Verification items for the finished model (mm, model axes). Face numbers are marked on the shaded views. Coordinates: 2 decimals unless noted, no trailing zeros. Order: outer loops, then holes, each group sorted by start corner. A loop starts at its lowest first (then second) coordinate and runs counter-clockwise, first axis right, second up. Notation, with made-up numbers: (-10.5, -21.75) -> (34.5, -21.75) arc R18 ccw to (34.5, -17.75) -> close; hole circle Ø5 at (2.25, -5.75). An arc over 180 degrees is marked (long way). Write item = value, one per line. Start each with the question number.
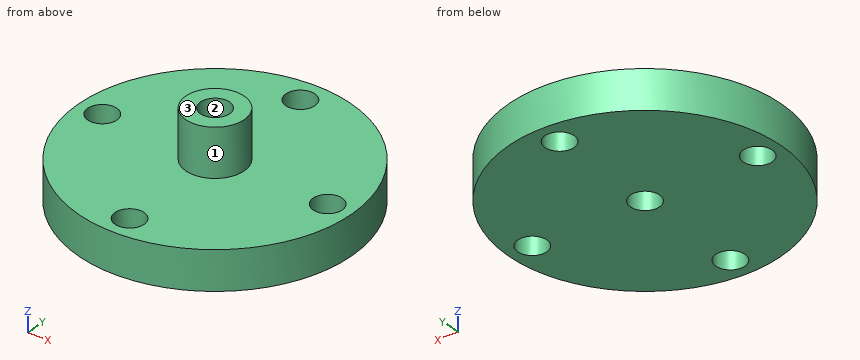
from build123d import *

# Parameters (mm, degrees)
SKETCH003_R   = 1.5
PAD003_DEPTH  = 8.9
SKETCH002_R   = 3
PAD002_DEPTH  = 4.9
SKETCH001_R   = 14
SKETCH001_R_2 = 1.5
PAD001_DEPTH  = 4


with BuildPart() as body003:
    # Sketch003 → Pad003 (new body)
    with BuildSketch(Plane.XY):
        Circle(SKETCH003_R)
    extrude(amount=PAD003_DEPTH)


with BuildPart() as body002:
    # Sketch002 (on DatumPlane) → Pad002 (new body)
    with BuildSketch(Plane.XY.offset(4)):
        Circle(SKETCH002_R)
    extrude(amount=PAD002_DEPTH)


with BuildPart() as cut:
    # Sketch001 → Pad001 (new body)
    with BuildSketch(Plane.XY):
        Circle(SKETCH001_R)
        with Locations((-11.5, 0)):
            Circle(SKETCH001_R_2, mode=Mode.SUBTRACT)
        with Locations((11.5, 0)):
            Circle(SKETCH001_R_2, mode=Mode.SUBTRACT)
        with Locations((0, 11.5)):
            Circle(SKETCH001_R_2, mode=Mode.SUBTRACT)
        with Locations((0, -11.5)):
            Circle(SKETCH001_R_2, mode=Mode.SUBTRACT)
    extrude(amount=PAD001_DEPTH)

    # Fusion: union Body002
    add(body002.part)

    # Cut: cut Body003
    add(body003.part, mode=Mode.SUBTRACT)


solid = cut.part
Item 1: Section check D-D (x = -11.5). Record the boundary of the cut face in (y, z).
Item 2: Section check C-C (z = 3.5). Record the boundary of the cut face in (x, y).
Item 3: Thickness scan on line 1 (Y direction, x = 0, z = 0.75); line 2 (Y direction, x = 0, z = 6.75); line 3 (Z direction, x = 7.75, y = -5.25). Record the ranges inside material, lowest first.
Item 4: Mould release check, pull along Y, two halves, no side actions. Record for the marked faces 1, 2 and 3: pulls with the +Y half, pulls with the -Y half, needs draft (parallel to the pull), parting line crosses it, or undercut.
Item 5: Section check A-A (x = 0). Record the boundary of the cut face in (y, z), then the cut area to 3 significant figures.
Item 6: Gauge pin test, flat ends, axial feed: P1, Ø5, axis at x = 11.5, y = 0, coming from the +Z side; P2, Ø3, axis at x = 3, z = 4.5, coming from the +Y side; P3, Ø1, axis at y = 3, z = 5.5, coming from the -X side. Record the tip position at first contact, or that the pin passes through.
Filled sheet:
q1.outline = (-7.98, 0) -> (-1.5, 0) -> (-1.5, 4) -> (-7.98, 4) -> close; (1.5, 0) -> (7.98, 0) -> (7.98, 4) -> (1.5, 4) -> close
q2.outline = circle Ø28 at (0, 0); hole circle Ø3 at (-11.5, 0); hole circle Ø3 at (0, -11.5); hole circle Ø3 at (0, 0); hole circle Ø3 at (0, 11.5); hole circle Ø3 at (11.5, 0)
q3.line_1 = -14 to -13, -10 to -1.5, 1.5 to 10, 13 to 14
q3.line_2 = -3 to -1.5, 1.5 to 3
q3.line_3 = 0 to 4
q4.face_1 = parting line crosses it
q4.face_2 = undercut
q4.face_3 = needs draft
q5.outline = (-14, 0) -> (-13, 0) -> (-13, 4) -> (-14, 4) -> close; (-10, 0) -> (-1.5, 0) -> (-1.5, 8.9) -> (-3, 8.9) -> (-3, 4) -> (-10, 4) -> close; (1.5, 0) -> (10, 0) -> (10, 4) -> (3, 4) -> (3, 8.9) -> (1.5, 8.9) -> close; (13, 0) -> (14, 0) -> (14, 4) -> (13, 4) -> close
q5.area = 90.7 mm^2
q6.P1 = 4
q6.P2 = 13.91
q6.P3 = -1.66
